```python
from build123d import *

# Parameters (mm, degrees)
SKETCH_1_R      = 1.6
SKETCH_1_R_2    = 0.45
EXTRUDE_1_DEPTH = 1.2
SKETCH_3_W      = 6
SKETCH_3_H      = 5
EXTRUDE_2_DEPTH = 2


with BuildPart() as part:
    # 草图1 → 凸台-拉伸1 (new body)
    with BuildSketch(Plane(origin=(0, 0, 0), x_dir=(1, 0, 0), z_dir=(0, 1, 0))):
        Polygon((19.25, -20.25), (21.25, -18.25), (21.25, 18.25), (19.25, 20.25), (-19.25, 20.25), (-21.25, 18.25), (-21.25, -18.25), (-19.25, -20.25), align=None)
        with Locations(Location((13.25, -12.25, 0), (0, 0, 270))):
            Circle(SKETCH_1_R, mode=Mode.SUBTRACT)
        with Locations(Location((-13.25, 12.25, 0), (0, 0, 270))):
            Circle(SKETCH_1_R, mode=Mode.SUBTRACT)
        with Locations(Location((-11.25, -13.25, 0), (0, 0, 270))):
            Circle(SKETCH_1_R_2, mode=Mode.SUBTRACT)
        with Locations(Location((-8.71, -13.25, 0), (0, 0, 270))):
            Circle(SKETCH_1_R_2, mode=Mode.SUBTRACT)
        with Locations(Location((-6.17, -13.25, 0), (0, 0, 270))):
            Circle(SKETCH_1_R_2, mode=Mode.SUBTRACT)
        with Locations(Location((-3.63, -13.25, 0), (0, 0, 270))):
            Circle(SKETCH_1_R_2, mode=Mode.SUBTRACT)
        with Locations(Location((-1.09, -13.25, 0), (0, 0, 270))):
            Circle(SKETCH_1_R_2, mode=Mode.SUBTRACT)
        with Locations(Location((1.45, -13.25, 0), (0, 0, 270))):
            Circle(SKETCH_1_R_2, mode=Mode.SUBTRACT)
        with Locations(Location((3.99, -13.25, 0), (0, 0, 270))):
            Circle(SKETCH_1_R_2, mode=Mode.SUBTRACT)
        with Locations(Location((6.53, -13.25, 0), (0, 0, 270))):
            Circle(SKETCH_1_R_2, mode=Mode.SUBTRACT)
        with Locations(Location((15.25, -3.25, 0), (0, 0, 270))):
            Circle(SKETCH_1_R_2, mode=Mode.SUBTRACT)
        with Locations(Location((15.25, -0.71, 0), (0, 0, 270))):
            Circle(SKETCH_1_R_2, mode=Mode.SUBTRACT)
        with Locations(Location((15.25, 1.83, 0), (0, 0, 270))):
            Circle(SKETCH_1_R_2, mode=Mode.SUBTRACT)
        with Locations(Location((15.25, 4.37, 0), (0, 0, 270))):
            Circle(SKETCH_1_R_2, mode=Mode.SUBTRACT)
    extrude(amount=EXTRUDE_1_DEPTH)

    # 草图3 → 凸台-拉伸2 (add)
    with BuildSketch(Plane(origin=(0, 1.2, 0), x_dir=(1, 0, 0), z_dir=(0, 1, 0))):
        with Locations((11.25, 9.75)):
            Rectangle(SKETCH_3_W, SKETCH_3_H)
    extrude(amount=EXTRUDE_2_DEPTH)


solid = part.part
```
Design review of the part built by this model. Coordinates are the model's own, in mm. A direction names the side the tool comes from. Round coordinates to 2 decimals unless told otherwise and drop trailing zeros. Write each loop counter-clockwise with the first axis right and the second up, starting at its lowest first coordinate (ties: lowest second). Pieces come first, ordered by that corner, then holes. Notation, with made-up numbers: (13.25, 74) -> (71.25, 74) arc R9 cw to (71.25, 78) -> close; hole circle Ø11 at (32, 51.25). An arc over 180 degrees is marked (long way). Answer in a Markdown table with one row per item.
Q1. Clearance check with flat-ended pins moving along their axes: pin 1 Ø1 at (y, z) = (2.5, -11) entering from +X; pin 2 Ø2.5 at (x, z) = (-13.25, -12.25) entering from +Y; pin 3 Ø12 at (x, z) = (8.5, 9) entering from +Y; pin 4 Ø0.6 at (x, y) = (12, 2) entering from -Z. State where each tip first meets the part, or that it passes through.
The answers:
| item | result |
|---|---|
| pin 1 | x = 14.25 |
| pin 2 | through |
| pin 3 | y = 1.2 |
| pin 4 | z = -12.25 |
Q2. Take a section at C-C, the plane y = 2.5. State the section outline as (x, z) points, then the cut area to 3 significant figures.
The answers:
| item | result |
|---|---|
| outline | (8.25, -12.25) -> (14.25, -12.25) -> (14.25, -7.25) -> (8.25, -7.25) -> close |
| area | 30.0 mm² |
Q3. Take a section at B-B, the plane x = -13.25. State the section outline as (y, z) points.
The answers:
| item | result |
|---|---|
| outline | (0, -20.25) -> (1.2, -20.25) -> (1.2, -13.85) -> (0, -13.85) -> close; (0, -10.65) -> (1.2, -10.65) -> (1.2, 20.25) -> (0, 20.25) -> close |
Q4. For faces 4 (the face through (15.696, 0.592, 3.191)), 5 (the face through (11, 2, -12.25)), 6 (the face through (14.25, 2, -10)), 7 (the face through (8.25, 2, -10)), list the 3-axis set-ups (+Z, -Z, +X, -X, +Y, -Y) from which the entire face can be reached by the end or side of a thin tool; tool diameter is ignored.
The answers:
| item | result |
|---|---|
| face 4 | +Y, -Y |
| face 5 | -Z, +X, -X, +Y |
| face 6 | +Z, -Z, +X, +Y |
| face 7 | +Z, -Z, -X, +Y |
Q5. To check wall thickness, follow L1, parallel to Y at x = -12.5, z = -0.5; L2, parallel to X at y = 0.3, z = 12.25; L3, parallel to X at y = 0.9, z = -1.83. State the ranges of each line that lie inside material, in increasing order. Write a range as [from, to].
The answers:
| item | result |
|---|---|
| L1 | [0, 1.2] |
| L2 | [-21.25, 11.65], [14.85, 21.25] |
| L3 | [-21.25, 14.8], [15.7, 21.25] |
Q6. Draft analysis for pull direction X (two halves, no side actions). For faces 1 (the face through (15.696, 0.592, -1.889)), 2 (the face through (20.2, 0.6, 19.3)), 3 (the face through (11, 3.2, -10)), state which applies: +X half, -X half, draft (parallel to the pull), parting line (faces both ways), or undercut.
The answers:
| item | result |
|---|---|
| face 1 | undercut |
| face 2 | +X half |
| face 3 | draft |
Q7. Take a section at A-A, the plane x = 13.25. State the section outline as (y, z) points.
The answers:
| item | result |
|---|---|
| outline | (0, -20.25) -> (1.2, -20.25) -> (1.2, -12.25) -> (3.2, -12.25) -> (3.2, -7.25) -> (1.2, -7.25) -> (1.2, 10.65) -> (0, 10.65) -> close; (0, 13.85) -> (1.2, 13.85) -> (1.2, 20.25) -> (0, 20.25) -> close |
